```python
from build123d import *

# Parameters (mm, degrees)
BOSS_EXTRUDE1_DEPTH     = 8
SKETCH2_R               = 1.55
CUT_EXTRUDE1_DEPTH      = 177
BOSS_EXTRUDE3_START     = 20.459902
SKETCH3_R               = 1.3
BOSS_EXTRUDE3_DEPTH     = 8
CUT_EXTRUDE2_START      = -2
CUT_EXTRUDE2_DEPTH      = 40
SKETCH3_3_R             = 1.3
CUT_EXTRUDE3_DEPTH      = 29.4599021
CUT_EXTRUDE3_DEPTH_BACK = 9
CUT_EXTRUDE4_DEPTH      = 6
CUT_EXTRUDE5_DEPTH      = 4.75
FILLET1_R               = 2


with BuildPart() as part:
    # Sketch1 → Boss-Extrude1 (new body)
    with BuildSketch(Plane.XY):
        with BuildLine():
            Line((-3, 0), (-3, 16.5))
            Line((-3, 16.5), (17, 16.5))
            ThreePointArc((17, 16.5), (85.039654136, 25.877266165), (153.079308271, 16.5))
            Line((153.079308271, 16.5), (173, 16.5))
            Line((173, 16.5), (173, 0.544153422))
            Line((173, 0.544153422), (173, -7.455846578))
            Line((173, -7.455846578), (170, -7.455846578))
            Line((170, -7.455846578), (170, 0))
            Line((170, 0), (170.005951762, 12.036791894))
            Line((170.005951762, 12.036791894), (170, 12))
            Line((170, 12), (167.5, 12))
            Line((167.5, 12), (167.5, 0))
            ThreePointArc((167.5, 0), (132.367862473, 14.191115036), (95, 20.459901787))
            Line((95, 20.459901787), (75, 20.459901787))
            ThreePointArc((75, 20.459901787), (37.632137527, 14.191115036), (2.5, 0))
            Line((2.5, 0), (2.5, 12))
            Line((2.5, 12), (0, 12))
            Line((0, 12), (0, 0))
            Line((0, 0), (0, -8))
            Line((0, -8), (-3, -8))
            Line((-3, -8), (-3, 0))
        make_face()
    extrude(amount=BOSS_EXTRUDE1_DEPTH)

    # Sketch2 → Cut-Extrude1 (cut, through all)
    with BuildSketch(Plane.ZY.offset(3)):
        with Locations((4, -4)):
            Circle(SKETCH2_R)
    extrude(amount=-CUT_EXTRUDE1_DEPTH, mode=Mode.SUBTRACT)

    # Sketch3 → Boss-Extrude3 (add)
    with BuildSketch(Plane(origin=(0, 0, 0), x_dir=(1, 0, 0), z_dir=(0, 1, 0)).offset(BOSS_EXTRUDE3_START)):
        Polygon((94, 17), (87, 17), (87, 29), (83, 29), (83, 17), (76, 17), (76, -8), (94, -8), align=None)
        with Locations((91, 14)):
            Circle(SKETCH3_R, mode=Mode.SUBTRACT)
        with Locations((79, -5)):
            Circle(SKETCH3_R, mode=Mode.SUBTRACT)
    extrude(amount=BOSS_EXTRUDE3_DEPTH)

    # Sketch5 → Cut-Extrude2 (cut)
    with BuildSketch(Plane.XY.offset(8).offset(CUT_EXTRUDE2_START)):
        with BuildLine():
            Line((82.9995, 25.459901787), (82.9995, 28.459901787))
            Line((82.9995, 28.459901787), (87.0005, 28.459901787))
            Line((87.0005, 28.459901787), (87.0005, 25.459901787))
            ThreePointArc((87.0005, 25.459901787), (85, 23.459401787), (82.9995, 25.459901787))
        make_face()
    extrude(amount=-CUT_EXTRUDE2_DEPTH, mode=Mode.SUBTRACT)

    # Sketch3<3> → Cut-Extrude3 (cut, two sides)
    with BuildSketch(Plane(origin=(0, 0, 0), x_dir=(1, 0, 0), z_dir=(0, 1, 0))) as cut_extrude3_sk:
        with Locations((79, -5)):
            Circle(SKETCH3_3_R)
    extrude(amount=CUT_EXTRUDE3_DEPTH, mode=Mode.SUBTRACT)
    extrude(cut_extrude3_sk.sketch, amount=-CUT_EXTRUDE3_DEPTH_BACK, mode=Mode.SUBTRACT)

    # Sketch6 → Cut-Extrude4 (cut)
    with BuildSketch(Plane(origin=(0, 28.459901787, 0), x_dir=(1, 0, 0), z_dir=(0, 1, 0))):
        Polygon((81.7995, 9.38), (88.113465558, 11.808798865), (91.0245, -3.288104906), (87.9495, -6), (81.7995, -6), align=None)
    extrude(amount=-CUT_EXTRUDE4_DEPTH, mode=Mode.SUBTRACT)

    # Sketch7 → Cut-Extrude5 (cut)
    with BuildSketch(Plane(origin=(0, 28.459901787, 0), x_dir=(1, 0, 0), z_dir=(0, 1, 0))):
        Polygon((91.0245, -3.288104906), (93.328799585, -8), (81.7995, -8), (81.7995, -6), (87.9495, -6), align=None)
    extrude(amount=-CUT_EXTRUDE5_DEPTH, mode=Mode.SUBTRACT)

    # Fillet1
    fillet1_edges = [part.edges().sort_by_distance(p)[0] for p in [
        (87, 22.937539816, -17),
        (83, 22.937539816, -17),
    ]]
    fillet(fillet1_edges, radius=FILLET1_R)


solid = part.part
```
Work out the finished part from the listing and answer in its coordinate system (mm). A direction names the side the tool comes from. Round coordinates to 2 decimals unless told otherwise and drop trailing zeros. Order: outer loops, then holes, each group sorted by start corner. A loop starts at its lowest first (then second) coordinate and runs counter-clockwise, first axis right, second up.
Q1. A tool of negligible diameter and unlimited length cuts with its end or side. For faces 1 (the flat face through (28, 14, 0)), 2 (the flat face through (7, 16.5, 4)), 3 (the flat face through (81.8, 26, -1)), 4 (the flat face through (88, 23.71, 7)), from which of +Z, -Z, +X, -X, +Y, -Y can it reach the whole face along a straight path? Write none if from no direction.
Solution:
face 1: -Z, -X, +Y, -Y
face 2: +Z, -Z, -X, +Y
face 3: +Y
face 4: +Z, +Y
Q2. A cutting plane is placed at C-C, the plane x = 85. Determine the outline of the cut face in (y, z).
Solution:
outline: (20.46, -29) - (23.46, -29) - (23.46, -10.61) - (22.46, -10.61) - (22.46, 6) - (23.71, 6) - (23.71, 8) - (20.46, 8) - close
Q3. The mould has two halves that part along Y. Classify faces 5 (the flat face through (83, 27, -14)), 6 (the flat face through (85, 22.46, -3)), 7 (the cylindrical face through (171.48, -3.93, 2.45)): pulls with the +Y half, pulls with the -Y half, needs draft (parallel to the pull), parting line crosses it, or undercut.
Solution:
face 5: needs draft
face 6: pulls with the +Y half
face 7: undercut
Q4. A cutting plane is placed at D-D, the plane y = 6. Determine the outline of the cut face in (x, z), then the cut area to 3 significant figures.
Solution:
outline: (-3, 0) - (0, 0) - (0, 8) - (-3, 8) - close; (2.5, 0) - (14.81, 0) - (14.81, 8) - (2.5, 8) - close; (155.19, 0) - (167.5, 0) - (167.5, 8) - (155.19, 8) - close; (170, 0) - (173, 0) - (173, 8) - (170, 8) - close
area: 245 mm2
Q5. Find the intervals of material crossed by line 1 along X through (y, z) = (3.5, 6.5); line 2 along X through (y, z) = (26.65, 5); line 3 along Y through (x, z) = (172.1, 4), in increasing order.
Solution:
line 1: x = -3 to 0, 2.5 to 9.38, 160.62 to 167.5, 170 to 173
line 2: x = 76 to 77.7, 80.3 to 81.8, 91.86 to 94
line 3: y = -7.46 to -5.55, -2.45 to 16.5
Q6. A cutting plane is placed at A-A, the plane y = -4. Determine the outline of the cut face in (x, z).
Solution:
outline: (-3, 0) - (0, 0) - (0, 2.45) - (-3, 2.45) - close; (-3, 5.55) - (0, 5.55) - (0, 8) - (-3, 8) - close; (170, 0) - (173, 0) - (173, 2.45) - (170, 2.45) - close; (170, 5.55) - (173, 5.55) - (173, 8) - (170, 8) - close
Q7. Given pin 1 Ø9 at (y, z) = (25.5, -5.5) entering from -X; pin 2 Ø8 at (x, z) = (32, -1) entering from +Y; pin 3 Ø1.2 at (x, z) = (169, 2) entering from -Y, each flat-ended and moving along its own axis, determine where each tip first touches the part or whether it passes through.
Solution:
pin 1: stops at x = 76
pin 2: stops at y = 21.03
pin 3: stops at y = 12
Q8. A cutting plane is placed at B-B, the plane y = 14. Determine the outline of the cut face in (x, z).
Solution:
outline: (-3, 0) - (36.96, 0) - (36.96, 8) - (-3, 8) - close; (133.04, 0) - (173, 0) - (173, 8) - (133.04, 8) - close
